Part model, mm, in its own coordinate system. A direction names the side the tool comes from. Give positions to 0.01 mm unless a question says otherwise; leave off trailing zeros. Loops run counter-clockwise (first coordinate to the right, second up) from the corner with the lowest first, then second, coordinate; pieces in that order, holes last. Notation, with made-up numbers: (-14.5, 16.5) -> (-5.5, 16.5) arc R8 cw to (-5.5, 24.5) -> close; hole circle Ø5 at (50, 39.25). An arc over 180 degrees is marked (long way). One line per question, with ' | ' between items.
```python
from build123d import *

# Parameters (mm, degrees)
BOSS_EXTRUDE3_DEPTH = 2.5
SKETCH4_R           = 3.5
BOSS_EXTRUDE4_DEPTH = 2.5
SKETCH5_R           = 2.51
CUT_EXTRUDE1_DEPTH  = 2.5
CUT_EXTRUDE2_DEPTH  = 2.5
FILLET2_R           = 3
FILLET3_R           = 1


with BuildPart() as part:
    # Sketch3 → Boss-Extrude3 (new body)
    with BuildSketch(Plane(origin=(0, 0, 0), x_dir=(0, 0, -1), z_dir=(1, 0, 0))):
        with BuildLine():
            Line((-35.995221199, 38.670285512), (-35.995221199, 25.670285512))
            ThreePointArc((-35.995221199, 25.670285512), (-33.495221199, 23.170285512), (-30.995221199, 25.670285512))
            Line((-30.995221199, 25.670285512), (-30.995221199, 38.670285512))
            ThreePointArc((-30.995221199, 38.670285512), (-33.495221199, 41.170285512), (-35.995221199, 38.670285512))
        make_face()
    extrude(amount=BOSS_EXTRUDE3_DEPTH)

    # Sketch4 → Boss-Extrude4 (add)
    with BuildSketch(Plane(origin=(2.5, 0, 0), x_dir=(0, 0, -1), z_dir=(1, 0, 0))):
        with Locations((-33.495221199, 38.670285512)):
            Circle(SKETCH4_R)
        with Locations((-33.495221199, 25.670285512)):
            Circle(SKETCH4_R)
    extrude(amount=-BOSS_EXTRUDE4_DEPTH)

    # Sketch5 → Cut-Extrude1 (cut)
    with BuildSketch(Plane(origin=(2.5, 0, 0), x_dir=(0, 0, -1), z_dir=(1, 0, 0))):
        with Locations((-33.495221199, 38.670285512)):
            Circle(SKETCH5_R)
        with Locations((-33.495221199, 25.670285512)):
            Circle(SKETCH5_R)
    extrude(amount=-CUT_EXTRUDE1_DEPTH, mode=Mode.SUBTRACT)

    # Sketch8 → Cut-Extrude2 (cut)
    with BuildSketch(Plane(origin=(2.5, 0, 0), x_dir=(0, 0, -1), z_dir=(1, 0, 0))):
        Polygon((-35.395221199, 35.220795769), (-35.395221199, 29.119775254), (-33.991986481, 32.170285512), align=None)
        Polygon((-31.595221199, 35.220795769), (-31.595221199, 29.119775254), (-32.998455917, 32.170285512), align=None)
        with BuildLine():
            Line((-34.645221199, 35.220795769), (-33.495221199, 32.720795769))
            Line((-33.495221199, 32.720795769), (-32.345221199, 35.220795769))
            ThreePointArc((-32.345221199, 35.220795769), (-33.495221199, 35.034150271), (-34.645221199, 35.220795769))
        make_face()
        with BuildLine():
            Line((-33.495221199, 31.619775254), (-32.345221199, 29.119775254))
            ThreePointArc((-32.345221199, 29.119775254), (-33.495221199, 29.306420752), (-34.645221199, 29.119775254))
            Line((-34.645221199, 29.119775254), (-33.495221199, 31.619775254))
        make_face()
    extrude(amount=-CUT_EXTRUDE2_DEPTH, mode=Mode.SUBTRACT)

    # Fillet2
    fillet2_edges = [part.edges().sort_by_distance(p)[0] for p in [
        (1.25, 36.220795769, 35.995221199),
        (1.25, 36.220795769, 30.995221199),
        (1.25, 28.119775254, 35.995221199),
        (1.25, 28.119775254, 30.995221199),
    ]]
    fillet(fillet2_edges, radius=FILLET2_R)

    # Fillet3
    fillet3_edges = [part.edges().sort_by_distance(p)[0] for p in [
        (1.25, 32.170285512, 32.998455917),
        (1.25, 32.170285512, 33.991986481),
    ]]
    fillet(fillet3_edges, radius=FILLET3_R)


solid = part.part
```
1) Saw through at D-D (x = 2.15). Give the cut face in (y, z) (3 decimals), and give its area (3 significant figures).
Found:
outline: (27.536, 30.534) arc R3 cw to (29.134, 30.995) -> (35.206, 30.995) arc R3 cw to (36.805, 30.534) arc R3.5 ccw (long way) to (36.805, 36.457) arc R3 cw to (35.206, 35.995) -> (29.134, 35.995) arc R3 cw to (27.536, 36.457) arc R3.5 ccw (long way) to start; hole circle Ø5.02 at (25.67, 33.495); hole (29.12, 31.595) -> (35.221, 31.595) -> (32.588, 32.806) arc R1 ccw to (31.752, 32.806) -> close; hole (29.12, 32.345) -> (31.62, 33.495) -> (29.12, 34.645) arc R3.636 cw to start; hole (29.12, 35.395) -> (31.752, 34.184) arc R1 ccw to (32.588, 34.184) -> (35.221, 35.395) -> close; hole (32.721, 33.495) -> (35.221, 32.345) arc R3.636 cw to (35.221, 34.645) -> close; hole circle Ø5.02 at (38.67, 33.495) | area: 57.3 mm2
2) Pull direction Y, two halves, no side cores. Call faces 1 (the flat face through (2.5, 32.3, 33.5)), 2 (the cylindrical face through (1.232, 32.164, 34.093)), 3 (the flat face through (1, 32, 35.395)): pulls with the +Y half, pulls with the -Y half, needs draft (parallel to the pull), parting line crosses it, or undercut.
Found:
face 1: needs draft | face 2: undercut | face 3: undercut
3) Saw through at B-B (z = 31.25). Give the cut face in (x, y), and give its area (3 significant figures).
Found:
outline: (0, 22.99) -> (2.5, 22.99) -> (2.5, 24.55) -> (0, 24.55) -> close; (0, 26.79) -> (2.5, 26.79) -> (2.5, 37.55) -> (0, 37.55) -> close; (0, 39.79) -> (2.5, 39.79) -> (2.5, 41.36) -> (0, 41.36) -> close | area: 34.7 mm2
4) Pin check, flat tips, straight feed: P1, Ø0.8, axis at x = 1, y = 32, coming from the -Z side; P2, Ø4, axis at y = 38.67, z = 33.5, coming from the +X side; P3, Ø0.8, axis at x = 0.5, y = 32, coming from the +Z side. Stop position of each tip, or through.
Found:
P1: z = 31 | P2: through | P3: z = 36
5) Saw through at A-A (y = 27.25). Give the cut face in (x, z), and give its area (3 significant figures).
Found:
outline: (0, 30.37) -> (2.5, 30.37) -> (2.5, 31.54) -> (0, 31.54) -> close; (0, 35.45) -> (2.5, 35.45) -> (2.5, 36.62) -> (0, 36.62) -> close | area: 5.86 mm2
6) Drill centre lines: line 1 (Z direction, x = 1.65, y = 33.5); line 2 (Z direction, x = 0.45, y = 34.5); line 3 (Y direction, x = 0.2, z = 34). Where is each one in solid material? Low to high.
Found:
line 1: 31 to 31.6, 32.39 to 33.14, 33.85 to 34.6, 35.4 to 36 | line 2: 31 to 31.6, 31.93 to 32.68, 34.31 to 35.06, 35.4 to 36 | line 3: 22.21 to 23.21, 28.13 to 29.27, 30.52 to 33.82, 35.07 to 36.21, 41.13 to 42.13
7) Tool access for faces 4 (the flat face through (1.268, 30.418, 34.798)), 5 (the cylindrical face through (1.268, 36.05, 30.874)), 6 (the cylindrical face through (1.27, 28.31, 36.11)), 7 (the flat face through (0, 32.3, 33.5)): list every direction of +Z, -Z, +X, -X, +Y, -Y with a clear straight run to the whole face (end or side of a thin tool).
Found:
face 4: +X, -X | face 5: -Z, +X, -X | face 6: +Z, +X, -X | face 7: +Z, -Z, -X, +Y, -Y
8) Saw through at C-C (y = 30). Give the cut face in (x, z).
Found:
outline: (0, 31) -> (2.5, 31) -> (2.5, 31.6) -> (0, 31.6) -> close; (0, 32) -> (2.5, 32) -> (2.5, 32.75) -> (0, 32.75) -> close; (0, 34.24) -> (2.5, 34.24) -> (2.5, 34.99) -> (0, 34.99) -> close; (0, 35.4) -> (2.5, 35.4) -> (2.5, 36) -> (0, 36) -> close
